The listing builds one solid part. Answer for the finished solid, in the listing's coordinates (mm). A direction names the side the tool comes from. Give positions to 0.01 mm unless a question says otherwise; leave off trailing zeros. Loops run counter-clockwise (first coordinate to the right, second up) from the corner with the lowest first, then second, coordinate; pieces in that order, holes last. Notation, with made-up numbers: M 30.25,6 L 53.25,6 A13 ccw 53.25,14 Z; hole C 23.5,-10 d8. An arc over 180 degrees is marked long. Use one line per item in the form item = value. Start each with the question number.
1. Straight lines are drawn through the part: line 1 (Z direction, x = -7.5, y = 1); line 2 (Z direction, x = 0.25, y = 4.25); line 3 (X direction, y = -0.5, z = 9). For each, find the intervals that lie inside material, in ascending order. Write a range as from..to.
2. The mould has two halves that part along Y. Classify faces 3 (the face through (0, 0, 0.076)), 4 (the face through (8.65, 2.72, 63.41)): released by +Y, released by -Y, zero draft, split by the parting line, or undercut.
3. Each of these flat-tipped pins is pushed along its axis until it touches: pin 1 Ø5 at (x, y) = (3, -2) entering from +Z; pin 2 Ø10 at (y, z) = (5.5, 27.5) entering from -X; pin 3 Ø10 at (x, z) = (-6.5, 27) entering from +Y. Where does it stop, or does it pass through?
4. For faces 1 (the face through (8.65, 2.72, 29.39)), 2 (the face through (1, -1, 0.051)), determine the directions among +Z, -Z, +X, -X, +Y, -Y from which every point of the face is accessible in a straight line to the end or side of a thin tool.
5. The part is cut by section A-A (z = 12). Write down the section's boundary in (x, y), and give its area (3 significant figures).
from build123d import *

# Parameters (mm, degrees)
SKETCH1_R           = 9.0678
BOSS_EXTRUDE1_DEPTH = 65.024
SKETCH4_R           = 7.937216361
CUT_EXTRUDE1_DEPTH  = 0.0254
SKETCH5_R           = 7.759625111
CUT_EXTRUDE2_DEPTH  = 0.0254
SKETCH6_R           = 4.737479436
CUT_EXTRUDE3_DEPTH  = 0.0254
CUT_EXTRUDE4_DEPTH  = 0.0254


with BuildPart() as part:
    # Sketch1 → Boss-Extrude1 (new body)
    with BuildSketch(Plane.XY):
        Circle(SKETCH1_R)
    extrude(amount=BOSS_EXTRUDE1_DEPTH)

    # Sketch2 → Cut-Revolve9 (revolve, cut)
    with BuildSketch(Plane(origin=(0, 0, 0), x_dir=(0, 0, -1), z_dir=(1, 0, 0)), mode=Mode.PRIVATE) as cut_revolve9_sk:
        with BuildLine():
            Line((-61.980472201, 9.198093657), (-59.460775409, 9.198093657))
            ThreePointArc((-59.460775409, 9.198093657), (-60.720623805, 8.672006552), (-61.980472201, 9.198093657))
        make_face()
    revolve(cut_revolve9_sk.sketch.rotate(Axis((0, 0.04619124, -3.327942322), (0, 0, 1)), 130.442191922), axis=Axis((0, 0.04619124, -3.327942322), (0, 0, 1)), mode=Mode.SUBTRACT)

    # Sketch4 → Cut-Extrude1 (cut)
    with BuildSketch(Plane.XY.offset(65.024)):
        Circle(SKETCH4_R)
    extrude(amount=-CUT_EXTRUDE1_DEPTH, mode=Mode.SUBTRACT)

    # Sketch5 → Cut-Extrude2 (cut)
    with BuildSketch(Plane(origin=(0, 0, 0), x_dir=(-1, 0, 0), z_dir=(0, 0, -1))):
        Circle(SKETCH5_R)
    extrude(amount=-CUT_EXTRUDE2_DEPTH, mode=Mode.SUBTRACT)

    # Sketch6 → Cut-Extrude3 (cut)
    with BuildSketch(Plane(origin=(0, 0, 0.0254), x_dir=(-1, 0, 0), z_dir=(0, 0, -1))):
        Circle(SKETCH6_R)
    extrude(amount=-CUT_EXTRUDE3_DEPTH, mode=Mode.SUBTRACT)

    # Sketch7 → Cut-Extrude4 (cut)
    with BuildSketch(Plane(origin=(0, 0, 0.0508), x_dir=(-1, 0, 0), z_dir=(0, 0, -1))):
        Polygon((0.885352187, 0.786979722), (2.508497864, 0.786979722), (2.508497864, -0.541048559), (0.885352187, -0.541048559), (0.885352187, -1.942856189), (-0.664014141, -1.942856189), (-0.664014141, -0.541048559), (-2.115008003, -0.541048559), (-2.115008003, 0.786979722), (-0.664014141, 0.786979722), (-0.664014141, 2.090414887), (0.885352187, 2.090414887), align=None)
    extrude(amount=-CUT_EXTRUDE4_DEPTH, mode=Mode.SUBTRACT)


solid = part.part
Derived:
q1.line_1 = 0.03..65
q1.line_2 = 0.05..65
q1.line_3 = -9.05..9.05
q2.face_3 = undercut
q2.face_4 = split by the parting line
q3.pin_1 = 65
q3.pin_2 = -9.05
q3.pin_3 = 8.94
q4.face_1 = +Z, -Z
q4.face_2 = -Z
q5.outline = C 0,0 d18.14
q5.area = 258 mm2
